Autodesk Inventor part; units mm, degrees
ref_plane "YZ Plane" through (0, 0, 0) normal (1, 0, 0) x (0, 1, 0)
ref_plane "XZ Plane" through (0, 0, 0) normal (0, 1, 0) x (-1, 0, 0)
ref_plane "XY Plane" through (0, 0, 0) normal (0, 0, 1) x (1, 0, 0)
sketch "Sketch1" plane through (0, 0, 0) normal (0, 1, 0) x (-1, 0, 0)
  circle A0 centre (0, 0) radius 5
  dimension "d1" = 10
extrude "Extrusion1" add sketch "Sketch1" along normal blind 15
sketch "Sketch2" plane through (0, 15, 0) normal (0, 1, 0) x (1, 0, 0)
  circle A0 centre (0, 0) radius 2.5
  line L0 (0, 0) -> (-0.5, 0)
  line L1 (-0.5, 0) -> (-0.5, -2.4495)
  line L2 (-0.5, 0) -> (-0.5, 2.4495)
  line L3 (0, 0) -> (0, 2.5)
  line L4 (0.5, 0) -> (0.5, -2.4495)
  line L5 (0.5, 0) -> (0.5, 2.4495)
  dimension "d4" = 5
  dimension "d5" = 0.5
extrude "Extrusion2" cut sketch "Sketch2" against normal blind 10 contours A0 L4 L5 | A0 L2 L1
sketch "Sketch3" plane through (0, 0, 0) normal (0, -1, 0) x (1, 0, 0)
  circle A0 centre (0, 0) radius 10
  dimension "d8" = 20
extrude "Extrusion3" add sketch "Sketch3" along normal blind 10
sketch "Sketch5" plane through (0, -10, 0) normal (0, -1, 0) x (1, 0, 0)
  circle A0 centre (0, 0) radius 2.5
extrude "Extrusion4" cut sketch "Sketch5" against normal blind 5
sketch "Sketch6" plane through (0, 0, 0) normal (0, 0, 1) x (1, 0, 0)
  line L0 (-10, -10) -> (10, -10)
  line L1 (10, -10) -> (8, -10)
  line L2 (8, -10) -> (8, -5)
  line L3 (2.5359, -10) -> (4.5359, -10)
  line L4 (4.5359, -10) -> (4.5359, -5)
  line L5 (4.5359, -5) -> (8, -5)
  line L6 (8, -5) -> (4.5359, -7)
  line L7 (0, -15) -> (0, 20)
  point P0 (0, 0)
  dimension "d13" = 2
  dimension "d14" = 2
  dimension "d15" = 4
  dimension "d16" = 30
  dimension "d17" = 2
revolve "Revolution1" cut sketch "Sketch6" angle 30 about axis through (0, -10, 0) along (0, -1, 0) contours L4 L6 L2 L0
pattern_circular "Circular Pattern1" count 6 over 360 about axis through (0, -10, 0) along (0, 1, 0) of "Revolution1"
properties part number "pot başlık"
Geometry: final body of the model. Coordinates: model frame, mm. Coordinates: 2 decimals unless noted, no trailing zeros. Loops run counter-clockwise (first coordinate to the right, second up) from the corner with the lowest first, then second, coordinate; pieces in that order, holes last. Notation, with made-up numbers: (82, 37.5) - (103, 37.5) arc R19 ccw to (103, 48.5) - close; hole circle Ø11 at (46.25, 76). An arc over 180 degrees is marked (long way). Put each result on its own line as item: value. Start each with the question number.
Q1. Pull-direction query (Z, two-part tool) for faces 1 (the flat face through (6, -8, 0)), 2 (the flat face through (0, 15, 0)), 3 (the flat face through (5.407, -8.021, 3.122)), 4 (the cylindrical face through (1.08, 7.4, 4.88)); classes: released by +Z, released by -Z, zero draft, split by the parting line, or undercut.
Q2. Cut plane B-B, the plane y = -4.5. Return loops of the section in (x, z), and give its area (3 significant figures).
Q3. Cut plane A-A, the plane y = 7.75. Return loops of the section in (x, z).
Q4. Line query: line 1 (X direction, y = -8.75, z = 5.5); line 2 (Y direction, x = -6.75, z = 5.25); line 3 (Z direction, x = 0, y = -2). Output: solid intervals per line, ascending.
Q5. Pin query (flat end, axial travel): pin 1 Ø0.6 at (x, z) = (1.5, -1) entering from +Y; pin 2 Ø1.5 at (x, y) = (7.5, 10) entering from +Z; pin 3 Ø5.5 at (y, z) = (8.5, 0) entering from +X; pin 4 Ø1.5 at (y, z) = (-2.5, -3.5) entering from -X. Return the tip coordinate at first contact, or that it passes through.
Filled sheet:
1. face 1: undercut
1. face 2: zero draft
1. face 3: undercut
1. face 4: split by the parting line
2. outline: circle Ø20 at (0, 0)
2. area: 314 mm²
3. outline: circle Ø10 at (0, 0); hole (-0.5, -2.45) - (-0.5, 2.45) arc R2.5 ccw to start; hole (0.5, -2.45) arc R2.5 ccw to (0.5, 2.45) - close
4. line 1: -8.35 to -5.81, -3.18 to 0, 3.18 to 8.35
4. line 2: -10 to 0
4. line 3: -10 to 10
5. pin 1: y = 5
5. pin 2: through
5. pin 3: x = 5
5. pin 4: x = -9.61
